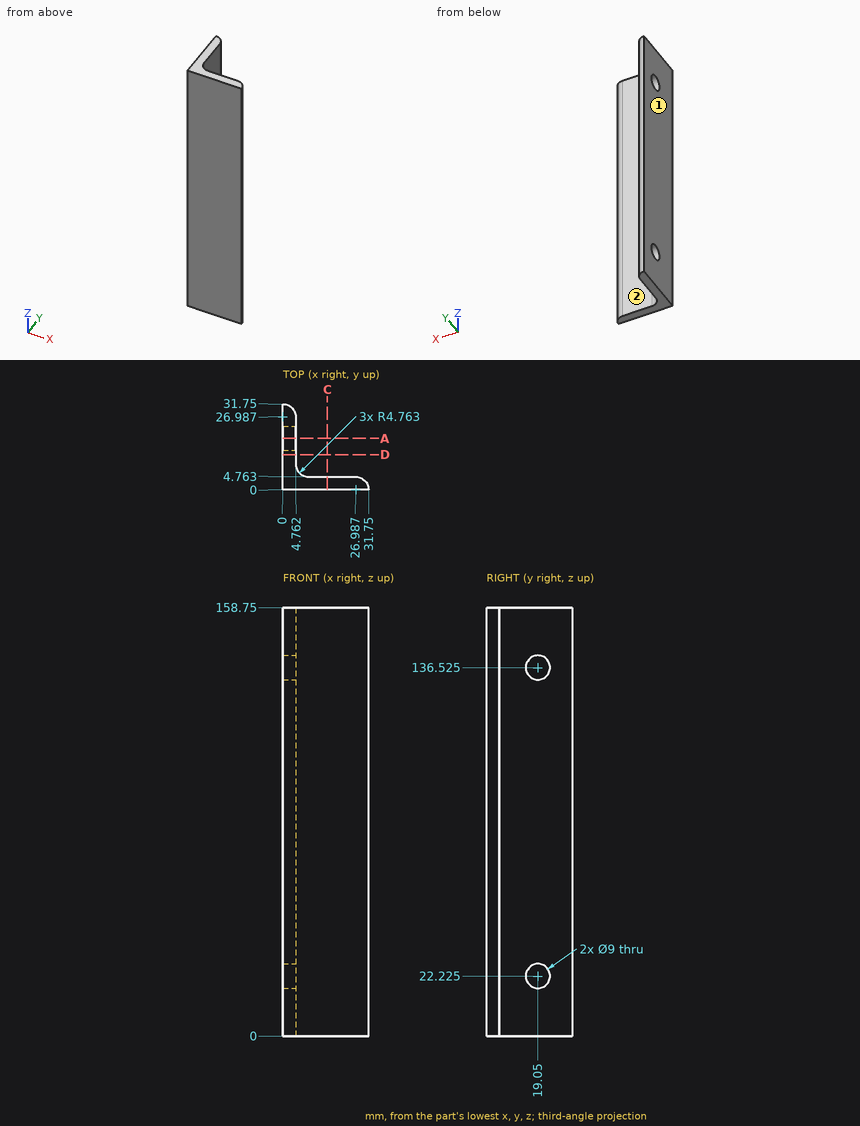
Part print with two shaded views. Sizes in mm from the minimum x, y, z corner. Round coordinates to 2 decimals unless told otherwise and drop trailing zeros. Loops run counter-clockwise (first coordinate to the right, second up) from the corner with the lowest first, then second, coordinate; pieces in that order, holes last.
1. Slice it at A-A (y = 19.05). Count the separate pieces of the cut face and the enclosed holes in it.
Solutions:
separate pieces: 3
enclosed holes: 0
2. Flat gauge pins, fed straight in: pin 1 (14 mm diameter, centred on x = 20, z = 118, fed in from +Y); pin 2 (10 mm diameter, centred on x = 12, y = 13, fed in from -Z); pin 3 (2 mm diameter, centred on y = 6.5, z = 133, fed in from +X); pin 4 (14 mm diameter, centred on y = 22, z = 101.5, fed in from +X). Where does each tip first touch, or does it go through?
Solutions:
pin 1: stops at y = 4.76
pin 2: passes through
pin 3: stops at x = 6.98
pin 4: stops at x = 4.76
3. Drill centre lines: line 1 along Y through (x, z) = (11, 114.5); line 2 along Y through (x, z) = (2.5, 21). Where is each one in solid material? Low to high.
Solutions:
line 1: y = 0 to 4.76
line 2: y = 0 to 14.72, 23.38 to 31.04
4. Two-plate mould, pull along X, no slides. Class the marked faces 1 and 2: pulls with the +X half, pulls with the -X half, needs draft (parallel to the pull), parting line crosses it, or undercut.
Solutions:
face 1: pulls with the -X half
face 2: needs draft
5. Slice it at C-C (x = 16.5). Give the cut face in (y, z).
Solutions:
outline: (0, 0) - (4.76, 0) - (4.76, 158.75) - (0, 158.75) - close
